Build history of the part. All positions in model axes, mm. Face numbers are marked on the shaded views. A direction names the side the tool comes from. Give positions to 0.01 mm unless a question says otherwise; leave off trailing zeros. Order: outer loops, then holes, each group sorted by start corner. A loop starts at its lowest first (then second) coordinate and runs counter-clockwise, first axis right, second up. Notation, with made-up numbers: M 48,47 L 67,47 A23 ccw 67,75 Z; hole C 14,-38 d4. An arc over 180 degrees is marked long. One line per item, written item: value.
from build123d import *

# Parameters (mm, degrees)
SKETCH1_R                   = 12.7
BOSS_EXTRUDE1_DEPTH         = 41.275
SKETCH3_R                   = 25.4
BOSS_EXTRUDE3_DEPTH         = 3.175
F_8_CLEARANCE_HOLE1_D       = 4.4958
F_20_8MMTOENDOFKEYWAY_DEPTH = 25
SKETCH8_R                   = 4.7625
BOSS_EXTRUDE4_DEPTH         = 15.875
FILLET1_R                   = 5


with BuildPart() as part:
    # Sketch1 → Boss-Extrude1 (new body)
    with BuildSketch(Plane(origin=(0, 0, 0), x_dir=(1, 0, 0), z_dir=(0, 1, 0))):
        Circle(SKETCH1_R)
    extrude(amount=BOSS_EXTRUDE1_DEPTH)

    # Sketch3 → Boss-Extrude3 (add)
    with BuildSketch(Plane.XZ):
        Circle(SKETCH3_R)
    extrude(amount=BOSS_EXTRUDE3_DEPTH)

    # #8 Clearance Hole1 (through all)
    with Locations(Plane(origin=(0, -3.175, 0), x_dir=(-1, 0, 0), z_dir=(0, -1, 0))):
        with Locations((0, 19.05), (-13.470384182, 13.470384182), (-19.05, 0), (-13.470384182, -13.470384182), (0, -19.05), (13.470384182, -13.470384182), (19.05, 0), (13.470384182, 13.470384182)):
            Hole(F_8_CLEARANCE_HOLE1_D / 2)

    # Sketch7 → 20.8mmToEndofKeyway (cut)
    with BuildSketch(Plane(origin=(0, 41.275, 0), x_dir=(1, 0, 0), z_dir=(0, 1, 0))):
        with BuildLine():
            Line((-2, 8.5), (2, 8.5))
            Line((2, 8.5), (2, 5.656854249))
            ThreePointArc((2, 5.656854249), (0, -6), (-2, 5.656854249))
            Line((-2, 5.656854249), (-2, 8.5))
        make_face()
    extrude(amount=-F_20_8MMTOENDOFKEYWAY_DEPTH, mode=Mode.SUBTRACT)

    # Sketch8 → Boss-Extrude4 (add)
    with BuildSketch(Plane.XZ.offset(3.175)):
        Circle(SKETCH8_R)
    extrude(amount=BOSS_EXTRUDE4_DEPTH)

    # Fillet1
    fillet1_edges = [part.edges().sort_by_distance(p)[0] for p in [
        (-4.7625, -3.175, 0),
    ]]
    fillet(fillet1_edges, radius=FILLET1_R)


solid = part.part
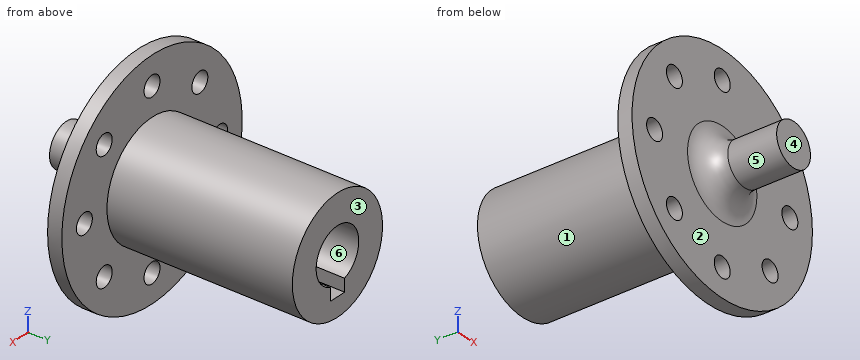
1) Mould opens along Z. For the marked faces 4, 5 and 6 say: released by +Z, released by -Z, zero draft, split by the parting line, or undercut.
Check values:
face 4: zero draft
face 5: split by the parting line
face 6: undercut
2) Tool access for the marked faces 1, 2 and 3: list every direction of +Z, -Z, +X, -X, +Y, -Y with a clear straight run to the whole face (end or side of a thin tool).
Check values:
face 1: +Y
face 2: -Y
face 3: +Z, -Z, +X, -X, +Y
3) Saw through at A-A, the plane x = 0. Give the number of separate pieces and of enclosed holes in the cut face, then the cut area to 3 significant figures.
Check values:
separate pieces: 3
enclosed holes: 0
area: 981 mm^2
4) Drill centre lines: probe 1 along X at (y, z) = (-2.35, 19.05); probe 2 along X at (y, z) = (33.5, 0); probe 3 along X at (y, z) = (-2, 2). Where is each one in solid material? Low to high. Write a range as from..to.
Check values:
probe 1: -16.8..-2.25, 2.25..16.8
probe 2: -12.7..-6, 6..12.7
probe 3: -25.32..-20.08, -18.02..18.02, 20.08..25.32
5) Saw through at B-B, the plane y = 20. Write the cut outline in (x, z).
Check values:
outline: C 0,0 d25.4; hole M -2,-8.5 L 2,-8.5 L 2,-5.66 A6 ccw long -2,-5.66 Z
6) Saw through at C-C, the plane x = 19. Write the cut outline in (y, z) (3 decimals).
Check values:
outline: M -3.175,-16.857 L 0,-16.857 L 0,-2.247 L -3.175,-2.247 Z; M -3.175,2.247 L 0,2.247 L 0,16.857 L -3.175,16.857 Z
7) Pin check, flat tips, straight feed: pin 1 (8 mm diameter, centred on x = 2.5, z = 0.5, fed in from +Y) (3 decimals); pin 2 (5 mm diameter, centred on x = 0, z = -19.05, fed in from -Y) (3 decimals); pin 3 (1.2 mm diameter, centred on x = -1, y = 33.5, fed in from +Z); pin 4 (3 mm diameter, centred on y = 35, z = -1.5, fed in from +X). Stop position of each tip, or through.
Check values:
pin 1: y = 41.275
pin 2: y = -3.175
pin 3: z = 12.69
pin 4: x = 12.7
